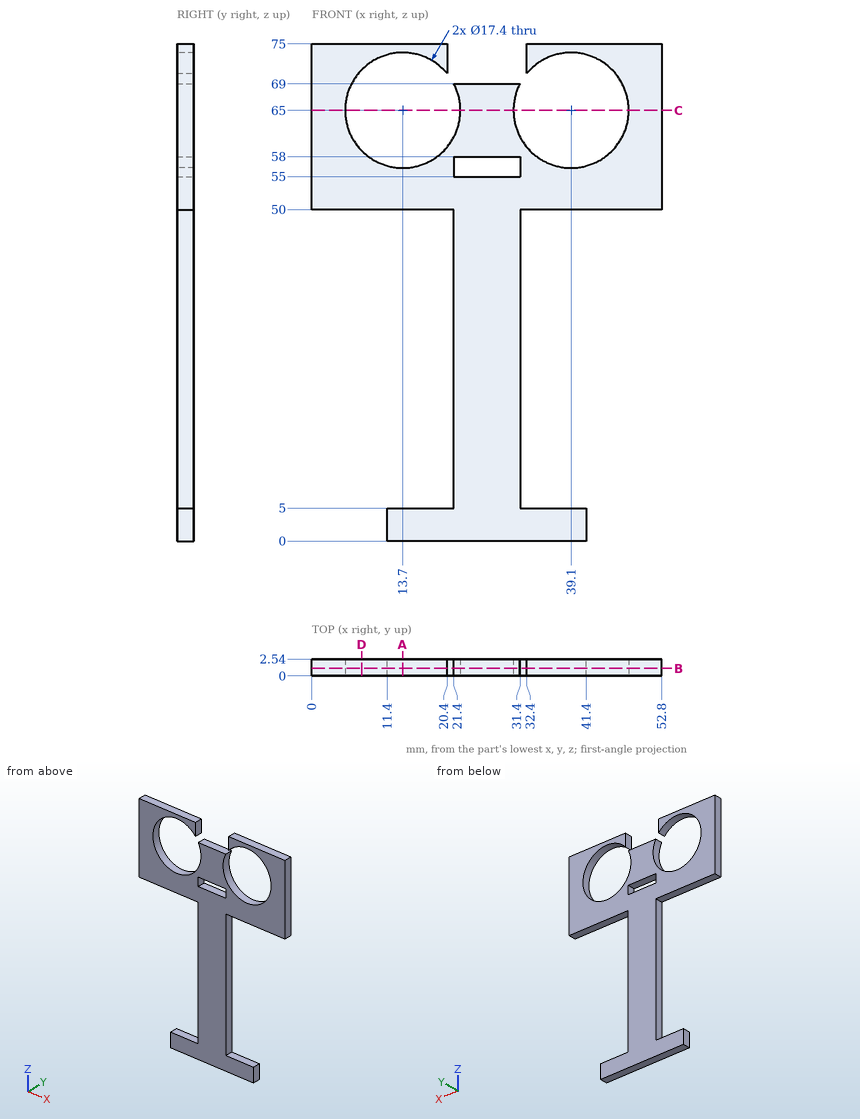
Design review of the part shown in the three views and the two pictorial views. Dimensions are in mm from the part's minimum x, y and z. Round coordinates to 2 decimals unless told otherwise and drop trailing zeros. Order: outer loops, then holes, each group sorted by start corner. A loop starts at its lowest first (then second) coordinate and runs counter-clockwise, first axis right, second up.
(1) Take a section at D-D, the plane x = 7.5. State the section outline as (y, z) points.
Working result:
outline: (0, 50) - (2.54, 50) - (2.54, 58.9) - (0, 58.9) - close; (0, 71.1) - (2.54, 71.1) - (2.54, 75) - (0, 75) - close
(2) Take a section at A-A, the plane x = 13.7. State the section outline as (y, z) points, plus the area to 3 significant figures.
Working result:
outline: (0, 0) - (2.54, 0) - (2.54, 5) - (0, 5) - close; (0, 50) - (2.54, 50) - (2.54, 56.3) - (0, 56.3) - close; (0, 73.7) - (2.54, 73.7) - (2.54, 75) - (0, 75) - close
area: 32.0 mm2
(3) Take a section at B-B, the plane y = 1.15. State the section outline as (x, z) points, plus the area to 3 significant figures.
Working result:
outline: (0, 50) - (21.4, 50) - (21.4, 5) - (11.4, 5) - (11.4, 0) - (41.4, 0) - (41.4, 5) - (31.4, 5) - (31.4, 50) - (52.8, 50) - (52.8, 75) - (32.4, 75) - (32.4, 70.55) arc R8.7 cw (long way) to (31.37, 69) - (21.43, 69) arc R8.7 cw (long way) to (20.4, 70.55) - (20.4, 75) - (0, 75) - close; hole (21.4, 55) - (31.4, 55) - (31.4, 58) - (21.4, 58) - close
area: 1,340 mm2
(4) Wall thickness on L1, parallel to Z at x = 39.1, y = 1.3; L2, parallel to X at y = 1, z = 65; L3, parallel to X at y = 1.65, z = 71: over which ranges is each line inside the solid? List them lowest first.
Working result:
L1: z = 0 to 5, 50 to 56.3, 73.7 to 75
L2: x = 0 to 5, 22.4 to 30.4, 47.8 to 52.8
L3: x = 0 to 7.4, 20 to 20.4, 32.4 to 32.8, 45.4 to 52.8
(5) Take a section at C-C, the plane z = 65. State the section outline as (x, y) points.
Working result:
outline: (0, 0) - (5, 0) - (5, 2.54) - (0, 2.54) - close; (22.4, 0) - (30.4, 0) - (30.4, 2.54) - (22.4, 2.54) - close; (47.8, 0) - (52.8, 0) - (52.8, 2.54) - (47.8, 2.54) - close
